```python
from build123d import *

# Parameters (mm, degrees)
F0_W      = 70
F0_H      = 36
F1_DEPTH  = 45
F2_W      = 59
F2_H      = 27
F3_DEPTH  = 40
F4_W      = 31.5
F4_H      = 27
F4_W_2    = 0.0242067426
F5_DEPTH  = 70.001
F6_R      = 1.25
F7_DEPTH  = 70.001
F9_DEPTH  = 2
F10_R     = 1.5
F11_DEPTH = 20
F12_R     = 2.05
F13_DEPTH = 25.4
F14_R     = 4
F14_R_2   = 2.05
F15_DEPTH = 2
F16_R     = 1


with BuildPart() as f1:
    # F0 (on Top) → F1 (new body)
    with BuildSketch(Plane.XY):
        Rectangle(F0_W, F0_H)
    extrude(amount=F1_DEPTH)

    # F2 (on face) → F3 (cut)
    with BuildSketch(Plane.XY.offset(45)):
        Rectangle(F2_W, F2_H)
    extrude(amount=-F3_DEPTH, mode=Mode.SUBTRACT)

    # F4 (on face) → F5 (cut, through all)
    with BuildSketch(Plane.YZ.offset(35)):
        with Locations((2.25, 31.5)):
            Rectangle(F4_W, F4_H)
        with Locations((18.0121033713, 31.5)):
            Rectangle(F4_W_2, F4_H)
    extrude(amount=-F5_DEPTH, mode=Mode.SUBTRACT)

    # F6 (on face) → F7 (cut, through all)
    with BuildSketch(Plane.YZ.offset(35)):
        with Locations((0, 12)):
            Circle(F6_R)
    extrude(amount=-F7_DEPTH, mode=Mode.SUBTRACT)

    # F8 (on face) → F9 (cut)
    with BuildSketch(Plane.XZ.offset(18)):
        Polygon((-28.0374098564, 0), (-21.9625901436, 0), (-23.4557936101, 2.6302886672), (-26.5057936101, 2.6524662959), (-28.05, 0.0221776287), align=None)
        Polygon((21.95, 0.0221776287), (21.9625901436, 0), (28.0374098564, 0), (26.5442063899, 2.6302886672), (23.4942063899, 2.6524662959), align=None)
    extrude(amount=-F9_DEPTH, mode=Mode.SUBTRACT)

    # F10 (on face) → F11 (cut)
    with BuildSketch(Plane.XZ.offset(16)):
        with BuildLine():
            Line((23.5, 0), (26.5, 0))
            ThreePointArc((26.5, 0), (25, 1.5), (23.5, 0))
        make_face()
        with BuildLine():
            ThreePointArc((23.5, 0), (25, -1.5), (26.5, 0))
            Line((26.5, 0), (23.5, 0))
        make_face()
        with Locations((-24.9706488103, 0)):
            Circle(F10_R)
    extrude(amount=-F11_DEPTH, mode=Mode.SUBTRACT)

    # F12 (on face) → F13 (cut)
    with BuildSketch(Plane.XZ.offset(18)):
        with Locations((-24.9807936101, 20)):
            Circle(F12_R)
        with Locations((25.0192063899, 20)):
            Circle(F12_R)
    extrude(amount=-F13_DEPTH, mode=Mode.SUBTRACT)

    # F14 (on face) → F15 (cut)
    with BuildSketch(Plane(origin=(0, -13.5, 0), x_dir=(-1, 0, 0), z_dir=(0, 1, 0))):
        with Locations((24.9807936101, 20)):
            Circle(F14_R)
        with Locations((24.9807936101, 20)):
            Circle(F14_R_2, mode=Mode.SUBTRACT)
        with Locations((-25.0192063899, 20)):
            Circle(F14_R)
        with Locations((-25.0192063899, 20)):
            Circle(F14_R_2, mode=Mode.SUBTRACT)
    extrude(amount=-F15_DEPTH, mode=Mode.SUBTRACT)

    # F16
    f16_edges = [f1.edges().sort_by_distance(p)[0] for p in [
        (0, -13.5, 45),
        (0, -18, 45),
    ]]
    fillet(f16_edges, radius=F16_R)


solid = f1.part
```
Geometry: final body of the model. Coordinates: model frame, mm. A direction names the side the tool comes from. Coordinates: 2 decimals unless noted, no trailing zeros. Order: outer loops, then holes, each group sorted by start corner. A loop starts at its lowest first (then second) coordinate and runs counter-clockwise, first axis right, second up. Notation, with made-up numbers: (-21, -21) -> (9, -21) arc R19 ccw to (9, 15) -> close; hole circle Ø5 at (2.25, 0.5). An arc over 180 degrees is marked (long way). Write item = value, one per line.
(1) Line query: line 1 (X direction, y = -17.3, z = 20); line 2 (Y direction, x = -5, z = 13); line 3 (Z direction, x = 33.3, y = 0). Output: solid intervals per line, ascending.
Solved:
line_1 = -35 to -27.03, -22.93 to 22.97, 27.07 to 35
line_2 = -18 to -13.5, 13.5 to 18
line_3 = 0 to 10.75, 13.25 to 18
(2) Cut plane D-D on z = 20. Return loops of the section in (x, y).
Solved:
outline = (-35, -18) -> (-27.03, -18) -> (-27.03, -15.5) -> (-28.98, -15.5) -> (-28.98, -13.5) -> (-35, -13.5) -> close; (-22.93, -18) -> (22.97, -18) -> (22.97, -15.5) -> (21.02, -15.5) -> (21.02, -13.5) -> (-20.98, -13.5) -> (-20.98, -15.5) -> (-22.93, -15.5) -> close; (27.07, -18) -> (35, -18) -> (35, -13.5) -> (29.02, -13.5) -> (29.02, -15.5) -> (27.07, -15.5) -> close
(3) Cut plane B-B on y = 0. Return loops of the section in (x, z), plus the area to 3 significant figures.
Solved:
outline = (-35, 0) -> (-26.47, 0) arc R1.5 cw to (-23.47, 0) -> (23.5, 0) arc R1.5 cw to (26.5, 0) -> (35, 0) -> (35, 10.75) -> (29.5, 10.75) -> (29.5, 5) -> (-29.5, 5) -> (-29.5, 10.75) -> (-35, 10.75) -> close; (-35, 13.25) -> (-29.5, 13.25) -> (-29.5, 18) -> (-35, 18) -> close; (29.5, 13.25) -> (35, 13.25) -> (35, 18) -> (29.5, 18) -> close
area = 458 mm²
(4) Cut plane C-C on x = 30.5. Return loops of the section in (y, z).
Solved:
outline = (-18, 0) -> (18, 0) -> (18, 18) -> (-13.5, 18) -> (-13.5, 44) arc R1 ccw to (-14.5, 45) -> (-17, 45) arc R1 ccw to (-18, 44) -> close; hole circle Ø2.5 at (0, 12)
(5) Pin query (flat end, axial travel): pin 1 Ø1.2 at (x, z) = (25, 0.5) entering from -Y; pin 2 Ø4 at (x, z) = (12.5, 32.5) entering from +Y; pin 3 Ø4 at (x, z) = (-26.5, 21) entering from +Y; pin 4 Ø2 at (y, z) = (0, 12) entering from +X. Return the tip coordinate at first contact, or that it passes through.
Solved:
pin_1 = 4
pin_2 = -13.5
pin_3 = -15.5
pin_4 = through
(6) Pull-direction query (X, two-part tool) for faces 1 (the flat face through (35, -4, 12)), 2 (the flat face through (0, 14, 18)), 3 (the flat face through (25, -16, 2)), 4 (the flat face through (27.3, -17, 1.3)); classes: pulls with the +X half, pulls with the -X half, needs draft (parallel to the pull), parting line crosses it, or undercut.
Solved:
face_1 = pulls with the +X half
face_2 = needs draft
face_3 = undercut
face_4 = undercut
(7) Cut plane A-A on z = 12. Return loops of the section in (x, y).
Solved:
outline = (-35, -18) -> (35, -18) -> (35, -1.25) -> (29.5, -1.25) -> (29.5, -13.5) -> (-29.5, -13.5) -> (-29.5, -1.25) -> (-35, -1.25) -> close; (-35, 1.25) -> (-29.5, 1.25) -> (-29.5, 13.5) -> (29.5, 13.5) -> (29.5, 1.25) -> (35, 1.25) -> (35, 18) -> (-35, 18) -> close
(8) Access query for faces 5 (the flat face through (0, -13.5, 24)), 6 (the flat face through (-22.7, -17, 1.3)), 7 (the flat face through (-35, -4, 12)), 8 (the flat face through (0, 18, 9)), 9 (the cylindrical face through (21.204, -14.486, 21.201)). Directions: +Z, -Z, +X, -X, +Y, -Y. A direction counts if a zero-diameter tool reaches every point of the face in a straight line with its end or side. Return the directions, or none.
Solved:
face_5 = +Z
face_6 = -Z, -Y
face_7 = +Z, -Z, -X, +Y, -Y
face_8 = +Z, -Z, +X, -X, +Y
face_9 = none
